```python
from build123d import *

# Parameters (mm, degrees)
CROQUIS2_W              = 50.8
CROQUIS2_H              = 6.31
CROQUIS3_W              = 50.8
CROQUIS3_H              = 6.31
CROQUIS4_W              = 60
CROQUIS4_H              = 53.155
SALIENTE_EXTRUIR1_DEPTH = 6.31
CROQUIS5_W              = 60
CROQUIS5_H              = 6.31
CORTAR_EXTRUIR1_DEPTH   = 6.31
CORTAR_EXTRUIR2_DEPTH   = 634
CROQUIS8_W              = 50.8
CROQUIS8_H              = 6.31
SALIENTE_EXTRUIR2_DEPTH = 63.5
CROQUIS9_R              = 5
CORTAR_EXTRUIR3_DEPTH   = 10
CROQUIS10_W             = 790.847933
CROQUIS10_H             = 6.31
CORTAR_EXTRUIR4_DEPTH   = 286
CROQUIS11_W             = 50.8
CROQUIS11_H             = 6.31
CROQUIS11_W_2           = 210
CORTAR_EXTRUIR5_DEPTH   = 13.11
CROQUIS12_W             = 50.8
CROQUIS12_H             = 6.31
SALIENTE_EXTRUIR3_DEPTH = 6.35
CROQUIS13_W             = 50.8
CROQUIS13_H             = 6.35
CORTAR_EXTRUIR6_DEPTH   = 6.35
CROQUIS14_W             = 85.847108528
CROQUIS14_H             = 473.639219469
CORTAR_EXTRUIR7_DEPTH   = 137
CROQUIS15_R             = 4.7625
CORTAR_EXTRUIR8_DEPTH   = 33
CROQUIS16_R             = 5
CORTAR_EXTRUIR9_DEPTH   = 33
CROQUIS18_R             = 4.7625
CORTAR_EXTRUIR10_DEPTH  = 50
CROQUIS19_W             = 50.8
CROQUIS19_H             = 6.31
SALIENTE_EXTRUIR4_DEPTH = 100


with BuildPart() as part:
    # Barrer1: sweep along a curve in space
    with BuildLine() as barrer1_path:
        Line((0, 0, 0), (0, -567.24, 0))
        Line((0, -567.24, 0), (0, -567.24, 336.2))
        Line((0, -567.24, 336.2), (1786.7, -567.24, 336.2))
        Line((1786.7, -567.24, 336.2), (1786.7, -567.24, 693.16))
        Line((1786.7, -567.24, 693.16), (1786.7, -436.23, 693.16))
        Line((1786.7, -436.23, 693.16), (1786.7, -436.23, 1487.162933))
    # Croquis2 → Barrer1 (sweep)
    with BuildSketch(Plane(origin=(0, 0, 0), x_dir=(1, 0, 0), z_dir=(0, 1, 0))):
        Rectangle(CROQUIS2_W, CROQUIS2_H)
        with Locations((210, 0)):
            Rectangle(CROQUIS2_W, CROQUIS2_H)
    sweep(path=barrer1_path.line, transition=Transition.RIGHT)

    # Barrer4: sweep along a curve in space
    with BuildLine() as barrer4_path:
        Line((-0.201028049, -3.155, -3.155), (-0.201028049, -3.155, -207.155))
        Line((-0.201028049, -3.155, -207.155), (-0.201028049, -53.155, -207.155))
    # Croquis3 → Barrer4 (sweep)
    with BuildSketch(Plane(origin=(0, 0, -3.155), x_dir=(-1, 0, 0), z_dir=(0, 0, -1))):
        with Locations((-210, -3.155)):
            Rectangle(CROQUIS3_W, CROQUIS3_H)
        with Locations((0, -3.155)):
            Rectangle(CROQUIS3_W, CROQUIS3_H)
    sweep(path=barrer4_path.line, transition=Transition.RIGHT)

    # Croquis4 → Saliente-Extruir1 (add)
    with BuildSketch(Plane(origin=(0, 0, -210.31), x_dir=(-1, 0, 0), z_dir=(0, 0, -1))):
        with Locations((-154.6, -26.5775)):
            Rectangle(CROQUIS4_W, CROQUIS4_H)
    extrude(amount=-SALIENTE_EXTRUIR1_DEPTH)

    # Croquis5 → Cortar-Extruir1 (cut)
    with BuildSketch(Plane.XY.offset(-204)):
        with Locations((154.6, -3.155)):
            Rectangle(CROQUIS5_W, CROQUIS5_H)
    extrude(amount=-CORTAR_EXTRUIR1_DEPTH, mode=Mode.SUBTRACT)

    # Croquis7 → Cortar-Extruir2 (cut)
    with BuildSketch(Plane(origin=(0, 0, 0), x_dir=(1, 0, 0), z_dir=(0, 1, 0))):
        Polygon((1761.3, -361.6), (2022.1, -361.6), (2022.1, 278.600557529), (-188.115947115, 278.600557529), (-188.115947115, -361.6), align=None)
    extrude(amount=-CORTAR_EXTRUIR2_DEPTH, mode=Mode.SUBTRACT)

    # Croquis8 → Saliente-Extruir2 (add)
    with BuildSketch(Plane(origin=(0, 0, 361.6), x_dir=(-1, 0, 0), z_dir=(0, 0, -1))):
        with Locations((-1786.7, -567.24)):
            Rectangle(CROQUIS8_W, CROQUIS8_H)
    extrude(amount=SALIENTE_EXTRUIR2_DEPTH)

    # Croquis9 → Cortar-Extruir3 (cut)
    with BuildSketch(Plane(origin=(0, -433.075, 0), x_dir=(1, 0, 0), z_dir=(0, 1, 0))):
        with Locations(Location((1786.7, -1454.162933, 0), (0, 0, 270))):
            Circle(CROQUIS9_R)
        with Locations(Location((1786.7, -1234.162933, 0), (0, 0, 270))):
            Circle(CROQUIS9_R)
        with Locations(Location((1996.7, -1234.162933, 0), (0, 0, 270))):
            Circle(CROQUIS9_R)
        with Locations(Location((1996.7, -1454.162933, 0), (0, 0, 270))):
            Circle(CROQUIS9_R)
    extrude(amount=-CORTAR_EXTRUIR3_DEPTH, mode=Mode.SUBTRACT)

    # Croquis10 → Cortar-Extruir4 (cut)
    with BuildSketch(Plane(origin=(2022.1, 0, 0), x_dir=(0, 0, -1), z_dir=(1, 0, 0))):
        with Locations((-1091.7389665, -436.23)):
            Rectangle(CROQUIS10_W, CROQUIS10_H)
    extrude(amount=-CORTAR_EXTRUIR4_DEPTH, mode=Mode.SUBTRACT)

    # Croquis11 → Cortar-Extruir5 (cut)
    with BuildSketch(Plane(origin=(0, -433.075, 0), x_dir=(1, 0, 0), z_dir=(0, 1, 0))):
        with Locations((1996.7, -693.16)):
            Rectangle(CROQUIS11_W, CROQUIS11_H)
        with Locations((1866.3, -693.16)):
            Rectangle(CROQUIS11_W_2, CROQUIS11_H)
    extrude(amount=-CORTAR_EXTRUIR5_DEPTH, mode=Mode.SUBTRACT)

    # Croquis12 → Saliente-Extruir3 (add)
    with BuildSketch(Plane(origin=(0, 0, 361.6), x_dir=(-1, 0, 0), z_dir=(0, 0, -1))):
        with Locations((-1996.7, -567.24)):
            Rectangle(CROQUIS12_W, CROQUIS12_H)
    extrude(amount=SALIENTE_EXTRUIR3_DEPTH)

    # Croquis13 → Cortar-Extruir6 (cut)
    with BuildSketch(Plane(origin=(0, -564.085, 0), x_dir=(1, 0, 0), z_dir=(0, 1, 0))):
        with Locations((1786.7, -301.275)):
            Rectangle(CROQUIS13_W, CROQUIS13_H)
    extrude(amount=-CORTAR_EXTRUIR6_DEPTH, mode=Mode.SUBTRACT)

    # Croquis14 → Cortar-Extruir7 (cut)
    with BuildSketch(Plane(origin=(0, -446.185, 0), x_dir=(1, 0, 0), z_dir=(0, 1, 0))):
        with Locations((1999.254154868, -571.717300183)):
            Rectangle(CROQUIS14_W, CROQUIS14_H)
    extrude(amount=-CORTAR_EXTRUIR7_DEPTH, mode=Mode.SUBTRACT)

    # Croquis15 → Cortar-Extruir8 (cut)
    with BuildSketch(Plane(origin=(0, -564.085, 0), x_dir=(1, 0, 0), z_dir=(0, 1, 0))):
        with Locations(Location((1786.7, -545.545, 0), (0, 0, 270))):
            Circle(CROQUIS15_R)
    extrude(amount=-CORTAR_EXTRUIR8_DEPTH, mode=Mode.SUBTRACT)

    # Croquis16 → Cortar-Extruir9 (cut)
    with BuildSketch(Plane(origin=(0, 0, 690.005), x_dir=(-1, 0, 0), z_dir=(0, 0, -1))):
        with Locations((-1786.7, -480.185)):
            Circle(CROQUIS16_R)
    extrude(amount=-CORTAR_EXTRUIR9_DEPTH, mode=Mode.SUBTRACT)

    # Croquis18 → Cortar-Extruir10 (cut)
    with BuildSketch(Plane(origin=(0, -570.395, 0), x_dir=(-1, 0, 0), z_dir=(0, -1, 0))):
        with Locations(Location((-1799.399999999, -342.552204666, 0), (0, 0, 90))):
            Circle(CROQUIS18_R)
        with Locations(Location((-1773.999999999, -317.152204666, 0), (0, 0, 90))):
            Circle(CROQUIS18_R)
    extrude(amount=-CORTAR_EXTRUIR10_DEPTH, mode=Mode.SUBTRACT)

    # Croquis19 → Saliente-Extruir4 (add)
    with BuildSketch(Plane(origin=(0, -446.185, 0), x_dir=(1, 0, 0), z_dir=(0, 1, 0))):
        with Locations((1786.7, -693.16)):
            Rectangle(CROQUIS19_W, CROQUIS19_H)
    extrude(amount=SALIENTE_EXTRUIR4_DEPTH)


solid = part.part
```
CAD build for the part. Positions are in the model's coordinates, mm. A direction names the side the tool comes from. Round coordinates to 2 decimals unless told otherwise and drop trailing zeros. Loops run counter-clockwise (first coordinate to the right, second up) from the corner with the lowest first, then second, coordinate; pieces in that order, holes last. Notation, with made-up numbers: M 56,-17.75 L 86,-17.75 A17 cw 86,3.25 Z; hole C 84.5,86 d10. An arc over 180 degrees is marked long. Use a Markdown table: item, result. Add a question column.
(1) Cut at B-B (y = -406). Give the cut face in (x, z) (3 decimals).
(2) Which spindle directions (+Z, -Z, +X, -X, +Y, -Y) get a long thin tool onto all of the face, cutting with end or side? Do faces 4 (the face through (1804.122, -567.284, 343.172)), 5 (the face through (1786, -457, 690.005)). Say none if no direction does.
(3) Cut at C-C (z = 613). Give the cut face in (x, y) (3 decimals).
(4) Flat gauge pins, fed straight in: pin 1 (4 mm diameter, centred on x = 1797, z = 623.5, fed in from +Y) (3 decimals); pin 2 (5.5 mm diameter, centred on x = 1774, z = 317.15, fed in from +Y). Where does each tip first touch, or does it go through?
(5) Cut at A-A (x = 1799.4). Give the cut face in (y, z) (3 decimals), and give its area (3 significant figures).
(6) Drill centre lines: line 1 (Z direction, x = 1774, y = -565) (3 decimals); line 2 (Z direction, x = 1781, y = -408) (3 decimals); line 3 (Y direction, x = 1779.5, z = 400) (3 decimals). Where is each one in solid material? Low to high.
(7) Pull direction Z, two halves, no side cores. Call faces 1 (the face through (1769.35, -567.28, 318.18)), 2 (the face through (1786, -460, 696.315)), 3 (the face through (1787, -564.085, 500)): +Z half, -Z half, draft (parallel to the pull), parting line (faces both ways), or undercut.
Geometry says:
| question | item | result |
|---|---|---|
| 1 | outline | M 1761.3,690.005 L 1812.1,690.005 L 1812.1,696.315 L 1761.3,696.315 Z |
| 2 | face 4 | +Y, -Y |
| 2 | face 5 | -Z, +X, -X, +Y |
| 3 | outline | M 1761.3,-570.395 L 1812.1,-570.395 L 1812.1,-564.085 L 1761.3,-564.085 Z |
| 4 | pin 1 | stops at y = -564.085 |
| 4 | pin 2 | passes through |
| 5 | outline | M -570.395,304.45 L -564.085,304.45 L -564.085,337.79 L -570.395,337.79 Z; M -570.395,347.315 L -564.085,347.315 L -564.085,690.005 L -346.185,690.005 L -346.185,696.315 L -570.395,696.315 Z |
| 5 | area | 3,790 mm² |
| 6 | line 1 | z = 304.45 to 312.39, 321.915 to 696.315 |
| 6 | line 2 | z = 690.005 to 696.315 |
| 6 | line 3 | y = -570.395 to -564.085 |
| 7 | face 1 | undercut |
| 7 | face 2 | +Z half |
| 7 | face 3 | draft |
